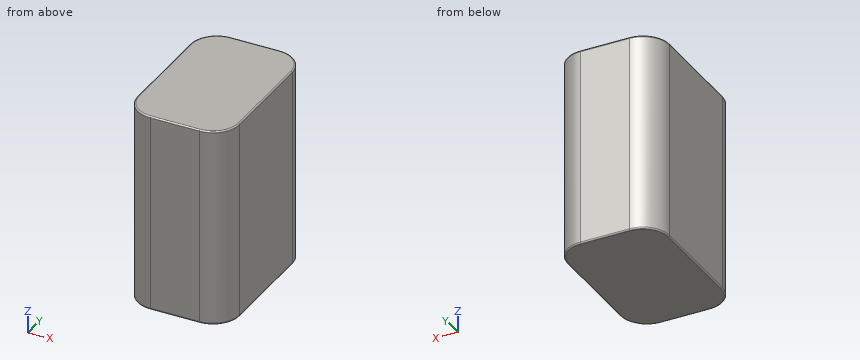
```python
from build123d import *

# Parameters (mm, degrees)
BOSS_EXTRUDE1_DEPTH = 0.75
BOSS_EXTRUDE2_START = 65
BOSS_EXTRUDE2_DEPTH = 65
BOSS_EXTRUDE3_START = 7.75
BOSS_EXTRUDE3_DEPTH = 7.75
FILLET1_R           = 0.5


with BuildPart() as part:
    # Sketch1 → Boss-Extrude1 (new body)
    with BuildSketch(Plane.XY):
        with BuildLine():
            Line((0, -28.25), (18, -28.25))
            ThreePointArc((18, -28.25), (24.894291117, -25.394291117), (27.75, -18.5))
            Line((27.75, -18.5), (27.75, 18.5))
            ThreePointArc((27.75, 18.5), (24.894291117, 25.394291117), (18, 28.25))
            Line((18, 28.25), (0, 28.25))
            ThreePointArc((0, 28.25), (-6.894291117, 25.394291117), (-9.75, 18.5))
            Line((-9.75, 18.5), (-9.75, -18.5))
            ThreePointArc((-9.75, -18.5), (-6.894291117, -25.394291117), (0, -28.25))
        make_face()
    extrude(amount=BOSS_EXTRUDE1_DEPTH)

    # Sketch2 → Boss-Extrude2 (add)
    with BuildSketch(Plane(origin=(0, 0, 0), x_dir=(-1, 0, 0), z_dir=(0, 0, -1)).offset(BOSS_EXTRUDE2_START)):
        with BuildLine():
            Line((0, 28.25), (-18, 28.25))
            ThreePointArc((-18, 28.25), (-24.894291117, 25.394291117), (-27.75, 18.5))
            Line((-27.75, 18.5), (-27.75, -18.5))
            ThreePointArc((-27.75, -18.5), (-24.894291117, -25.394291117), (-18, -28.25))
            Line((-18, -28.25), (0, -28.25))
            ThreePointArc((0, -28.25), (6.894291117, -25.394291117), (9.75, -18.5))
            Line((9.75, -18.5), (9.75, 18.5))
            ThreePointArc((9.75, 18.5), (6.894291117, 25.394291117), (0, 28.25))
        make_face()
        with BuildLine():
            Line((-27, 18), (-27, -18))
            ThreePointArc((-27, -18), (-24.363961031, -24.363961031), (-18, -27))
            Line((-18, -27), (0, -27))
            ThreePointArc((0, -27), (6.363961031, -24.363961031), (9, -18))
            Line((9, -18), (9, 18))
            ThreePointArc((9, 18), (6.363961031, 24.363961031), (0, 27))
            Line((0, 27), (-18, 27))
            ThreePointArc((-18, 27), (-24.363961031, 24.363961031), (-27, 18))
        make_face(mode=Mode.SUBTRACT)
    extrude(amount=-BOSS_EXTRUDE2_DEPTH)

    # Sketch3 → Boss-Extrude3 (add)
    with BuildSketch(Plane(origin=(0, 0, -65), x_dir=(-1, 0, 0), z_dir=(0, 0, -1)).offset(BOSS_EXTRUDE3_START)):
        with BuildLine():
            Line((9.75, -18.5), (9.75, 18.5))
            ThreePointArc((9.75, 18.5), (6.894291117, 25.394291117), (0, 28.25))
            Line((0, 28.25), (-18, 28.25))
            ThreePointArc((-18, 28.25), (-24.894291117, 25.394291117), (-27.75, 18.5))
            Line((-27.75, 18.5), (-27.75, -18.5))
            ThreePointArc((-27.75, -18.5), (-24.894291117, -25.394291117), (-18, -28.25))
            Line((-18, -28.25), (0, -28.25))
            ThreePointArc((0, -28.25), (6.894291117, -25.394291117), (9.75, -18.5))
        make_face()
    extrude(amount=-BOSS_EXTRUDE3_DEPTH)

    # Fillet1
    fillet1_edges = [part.edges().sort_by_distance(p)[0] for p in [
        (-6.894291117, -25.394291117, 0.75),
        (9, -28.25, 0.75),
        (24.894291117, -25.394291117, 0.75),
        (27.75, 0, 0.75),
        (24.894291117, 25.394291117, 0.75),
        (9, 28.25, 0.75),
        (-6.894291117, 25.394291117, 0.75),
        (9, -28.25, -72.75),
        (-6.894291117, -25.394291117, -72.75),
        (-9.75, 0, -72.75),
        (-6.894291117, 25.394291117, -72.75),
        (9, 28.25, -72.75),
        (24.894291117, 25.394291117, -72.75),
        (27.75, 0, -72.75),
        (24.894291117, -25.394291117, -72.75),
        (-9.75, 0, 0.75),
    ]]
    fillet(fillet1_edges, radius=FILLET1_R)


solid = part.part
```
Verification items for the finished model (mm, model axes). Round coordinates to 2 decimals unless told otherwise and drop trailing zeros. Write each loop counter-clockwise with the first axis right and the second up, starting at its lowest first coordinate (ties: lowest second). Pieces come first, ordered by that corner, then holes.
1. Section check B-B on z = -49.5. Enter the section's corners in (x, y).
2. Section check C-C on x = 2.5. Enter the section's corners in (y, z), plus the area to 3 significant figures.
3. Scan lines: L1, parallel to Z at x = 19, y = -16.5; L2, parallel to X at y = 9.5, z = -49.5; L3, parallel to Y at x = 9.5, z = -3. Record each from-to range of solid material in increasing order.
4. Section check A-A on y = 2.5. Enter the section's corners in (x, z).
Answer:
1. outline: (-9.75, -18.5) arc R9.75 ccw to (0, -28.25) - (18, -28.25) arc R9.75 ccw to (27.75, -18.5) - (27.75, 18.5) arc R9.75 ccw to (18, 28.25) - (0, 28.25) arc R9.75 ccw to (-9.75, 18.5) - close; hole (-9, -18) arc R9 ccw to (0, -27) - (18, -27) arc R9 ccw to (27, -18) - (27, 18) arc R9 ccw to (18, 27) - (0, 27) arc R9 ccw to (-9, 18) - close
2. outline: (-28.25, -72.25) arc R0.5 ccw to (-27.75, -72.75) - (27.75, -72.75) arc R0.5 ccw to (28.25, -72.25) - (28.25, 0.25) arc R0.5 ccw to (27.75, 0.75) - (-27.75, 0.75) arc R0.5 ccw to (-28.25, 0.25) - close; hole (-27, -65) - (27, -65) - (27, 0) - (-27, 0) - close
2. area: 643 mm2
3. L1: z = -72.75 to -65, 0 to 0.75
3. L2: x = -9.75 to -9, 27 to 27.75
3. L3: y = -28.25 to -27, 27 to 28.25
4. outline: (-9.75, -72.25) arc R0.5 ccw to (-9.25, -72.75) - (27.25, -72.75) arc R0.5 ccw to (27.75, -72.25) - (27.75, 0.25) arc R0.5 ccw to (27.25, 0.75) - (-9.25, 0.75) arc R0.5 ccw to (-9.75, 0.25) - close; hole (-9, -65) - (27, -65) - (27, 0) - (-9, 0) - close
